```python
from build123d import *

# Parameters (mm, degrees)
P_IDAT_VYSUNUT_M1_DEPTH  = 4.7
P_IDAT_VYSUNUT_M2_DEPTH  = 4.7
SKICA3_R                 = 2.425
ODEBRAT_VYSUNUT_M1_DEPTH = 14.6
P_IDAT_VYSUNUT_M3_DEPTH  = 4
SKICA5_R                 = 3
ODEBRAT_VYSUNUT_M2_DEPTH = 1.6
SKETCH1_R                = 2.2
CUT_EXTRUDE1_DEPTH       = 3


with BuildPart() as part:
    # Skica1 → Přidat vysunutím1 (new body)
    with BuildSketch(Plane.XY):
        with BuildLine():
            Line((3.15, 0), (23.94, 0))
            ThreePointArc((23.94, 0), (26.167386361, 0.922613639), (27.09, 3.15))
            Line((27.09, 3.15), (27.09, 34))
            Line((27.09, 34), (0, 34))
            Line((0, 34), (0, 3.15))
            ThreePointArc((0, 3.15), (0.922613639, 0.922613639), (3.15, 0))
        make_face()
    extrude(amount=P_IDAT_VYSUNUT_M1_DEPTH)

    # Skica2 → Přidat vysunutím2 (add)
    with BuildSketch(Plane(origin=(0, 0, 0), x_dir=(-1, 0, 0), z_dir=(0, 0, -1))):
        Polygon((-9.71157467, 33.71157467), (-0.024211768, 24.024211768), (14.825030637, 38.873454173), (5.137667735, 48.560817075), align=None)
        Polygon((-41.915030637, 38.873454173), (-27.065788232, 24.024211768), (-17.37842533, 33.71157467), (-32.227667735, 48.560817075), align=None)
    extrude(amount=-P_IDAT_VYSUNUT_M2_DEPTH)

    # Skica3 → Odebrat vysunutím1 (cut)
    with BuildSketch(Plane.XY.offset(4.7)):
        with Locations((5.575, 29.575)):
            Circle(SKICA3_R)
        with Locations((13.545, 29.575)):
            Circle(SKICA3_R)
        with Locations((21.515, 29.575)):
            Circle(SKICA3_R)
        with Locations((5.575, 21.605)):
            Circle(SKICA3_R)
        with Locations((13.545, 21.605)):
            Circle(SKICA3_R)
        with Locations((21.515, 21.605)):
            Circle(SKICA3_R)
        with Locations((21.515, 13.635)):
            Circle(SKICA3_R)
        with Locations((13.545, 13.635)):
            Circle(SKICA3_R)
        with Locations((5.575, 13.635)):
            Circle(SKICA3_R)
        with Locations((5.575, 5.665)):
            Circle(SKICA3_R)
        with Locations((13.545, 5.665)):
            Circle(SKICA3_R)
        with Locations((21.515, 5.665)):
            Circle(SKICA3_R)
    extrude(amount=-ODEBRAT_VYSUNUT_M1_DEPTH, mode=Mode.SUBTRACT)

    # Skica4 → Přidat vysunutím3 (add)
    with BuildSketch(Plane.XY.offset(4.7)):
        Polygon((-5.137667735, 48.560817075), (9.069595949, 34.353553391), (8.362489168, 33.646446609), (-5.844774516, 47.853710294), align=None)
        Polygon((32.227667735, 48.560817075), (18.020404051, 34.353553391), (18.727510832, 33.646446609), (32.934774516, 47.853710294), align=None)
        Polygon((-14.825030637, 38.873454173), (0, 24.048423535), (0.707106781, 24.755530317), (-14.117923856, 39.580560954), align=None)
        Polygon((41.915030637, 38.873454173), (27.09, 24.048423535), (26.382893219, 24.755530317), (41.207923856, 39.580560954), align=None)
    extrude(amount=P_IDAT_VYSUNUT_M3_DEPTH)

    # Skica5 → Odebrat vysunutím2 (cut)
    with BuildSketch(Plane(origin=(0, 0, 0), x_dir=(-1, 0, 0), z_dir=(0, 0, -1))):
        with Locations((-21.515, 29.575)):
            Circle(SKICA5_R)
        with Locations((-13.545, 29.575)):
            Circle(SKICA5_R)
        with Locations((-5.575, 29.575)):
            Circle(SKICA5_R)
        with Locations((-5.575, 21.605)):
            Circle(SKICA5_R)
        with Locations((-13.545, 21.605)):
            Circle(SKICA5_R)
        with Locations((-21.515, 21.605)):
            Circle(SKICA5_R)
        with Locations((-13.545, 5.665)):
            Circle(SKICA5_R)
        with Locations((-21.515, 5.665)):
            Circle(SKICA5_R)
        with Locations((-5.575, 5.665)):
            Circle(SKICA5_R)
        with Locations((-5.575, 13.635)):
            Circle(SKICA5_R)
        with Locations((-13.545, 13.635)):
            Circle(SKICA5_R)
        with Locations((-21.515, 13.635)):
            Circle(SKICA5_R)
    extrude(amount=-ODEBRAT_VYSUNUT_M2_DEPTH, mode=Mode.SUBTRACT)

    # Sketch1 → Cut-Extrude1 (cut)
    with BuildSketch(Plane.XY.offset(4.7)):
        with Locations((-6.09226189, 39.828048327)):
            Circle(SKETCH1_R)
        with Locations((33.18226189, 39.828048327)):
            Circle(SKETCH1_R)
    extrude(amount=-CUT_EXTRUDE1_DEPTH, mode=Mode.SUBTRACT)


solid = part.part
```
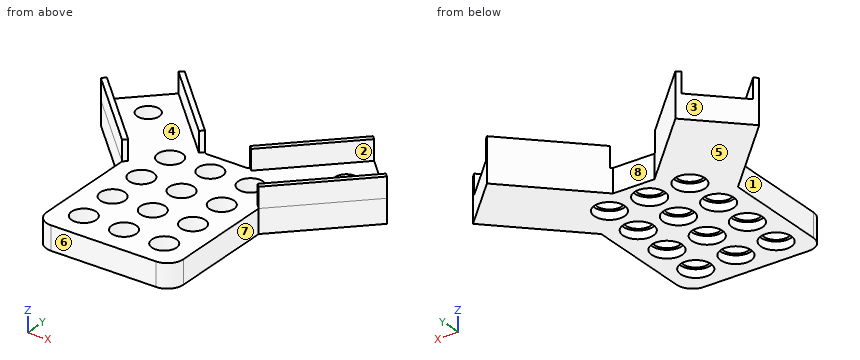
CAD build for the part. Positions are in the model's coordinates, mm. Face numbers are marked on the shaded views. A direction names the side the tool comes from. Round coordinates to 2 decimals unless told otherwise and drop trailing zeros. Order: outer loops, then holes, each group sorted by start corner. A loop starts at its lowest first (then second) coordinate and runs counter-clockwise, first axis right, second up. Notation, with made-up numbers: (18.25, 65) - (68.25, 65) arc R25 ccw to (68.25, 90) - close; hole circle Ø11 at (17, -34). An arc over 180 degrees is marked (long way). Answer in a Markdown table with one row per item. Add a question column.
(1) Band-saw the part on D-D on y = 4. List the corners of the cut face in (x, z).
(2) Probe L1, parallel to X at y = 5.5, z = 4; L2, parallel to X at y = 22.5, z = 4.25; L3, parallel to Y at x = 3.5, z = 4.5. List the from-to ranges inside material, lowest first. Write a range as [from, to].
(3) Band-saw the part on A-A on z = 7.75. List the corners of the cut face in (x, y), and give its area (3 significant figures).
(4) Mould opens along Y. For the marked faces 1, 2 and 3 say: +Y half, -Y half, draft (parallel to the pull), parting line (faces both ways), or undercut.
(5) Drop flat-ended pins along their axis: pin 1 Ø4.5 at (x, y) = (13.545, 5.665) entering from +Z; pin 2 Ø4 at (x, y) = (33.18, 39.83) entering from +Z; pin 3 Ø6.5 at (x, y) = (21.515, 29.575) entering from +Z; pin 4 Ø3 at (y, z) = (19.5, 4.5) entering from -X. Give the stop position or say it passes through.
(6) 3-axis set-ups, long thin cutter, end or side, ignore diameter. For the marked faces 4, 5, 6, 7 and 8: which of +Z, -Z, +X, -X, +Y, -Y reach the whole face in a straight line?
(7) Band-saw the part on C-C on z = 3. Count the separate pieces of the cut face and the enclosed holes in it, and give its area (3 significant figures).
(8) Band-saw the part on B-B on y = 37. List the corners of the cut face in (x, z).
Data:
| question | item | result |
|---|---|---|
| 1 | outline | (0, 0) - (3.08, 0) - (3.08, 1.6) - (3.81, 1.6) - (3.81, 4.7) - (0, 4.7) - close; (7.34, 1.6) - (8.07, 1.6) - (8.07, 0) - (11.05, 0) - (11.05, 1.6) - (11.78, 1.6) - (11.78, 4.7) - (7.34, 4.7) - close; (15.31, 1.6) - (16.04, 1.6) - (16.04, 0) - (19.02, 0) - (19.02, 1.6) - (19.75, 1.6) - (19.75, 4.7) - (15.31, 4.7) - close; (23.28, 1.6) - (24.01, 1.6) - (24.01, 0) - (27.09, 0) - (27.09, 4.7) - (23.28, 4.7) - close |
| 2 | L1 | x = [0, 3.16], [7.99, 11.13], [15.96, 19.1], [23.93, 27.09] |
| 2 | L2 | x = [0, 3.32], [7.83, 11.29], [15.8, 19.26], [23.77, 27.09] |
| 2 | L3 | y = [0, 4.41], [6.92, 12.38], [14.89, 20.35], [22.86, 28.32], [30.83, 39.92] |
| 3 | outline | (-14.83, 38.87) - (0, 24.05) - (0.71, 24.76) - (-14.12, 39.58) - close; (-5.84, 47.85) - (8.36, 33.65) - (9.07, 34.35) - (-5.14, 48.56) - close; (18.02, 34.35) - (18.73, 33.65) - (32.93, 47.85) - (32.23, 48.56) - close; (26.38, 24.76) - (27.09, 24.05) - (41.92, 38.87) - (41.21, 39.58) - close |
| 3 | area | 82.1 mm^2 |
| 4 | face 1 | draft |
| 4 | face 2 | undercut |
| 4 | face 3 | +Y half |
| 5 | pin 1 | passes through |
| 5 | pin 2 | stops at z = 1.7 |
| 5 | pin 3 | stops at z = 4.7 |
| 5 | pin 4 | stops at x = 0 |
| 6 | face 4 | +Z |
| 6 | face 5 | -Z, +X, -X, +Y, -Y |
| 6 | face 6 | +Z, -Z, +X, -X, -Y |
| 6 | face 7 | +Z, -Z, +X, -Y |
| 6 | face 8 | +Z, -Z, +Y |
| 7 | separate pieces | 1 |
| 7 | enclosed holes | 14 |
| 7 | area | 1,140 mm^2 |
| 8 | outline | (-12.95, 0) - (6.42, 0) - (6.42, 8.7) - (5.01, 8.7) - (5.01, 4.7) - (-11.54, 4.7) - (-11.54, 8.7) - (-12.95, 8.7) - close; (20.67, 0) - (40.04, 0) - (40.04, 8.7) - (38.63, 8.7) - (38.63, 4.7) - (22.08, 4.7) - (22.08, 8.7) - (20.67, 8.7) - close |
